Build history of the part. All positions in model axes, mm. A direction names the side the tool comes from. Coordinates: 2 decimals unless noted, no trailing zeros. Write each loop counter-clockwise with the first axis right and the second up, starting at its lowest first coordinate (ties: lowest second). Pieces come first, ordered by that corner, then holes.
Autodesk Fusion 360 part; units mm, degrees
sketch "Sketch1" plane through (0, 0, 0) normal (0, 1, 0) x (1, 0, 0) in component "[a]_belt_clamp_x2"
  line L0 (4.25, 7.875) -> (-4.25, 7.875)
  line L1 (-4.25, 7.875) -> (-4.25, -7.875)
  line L2 (-4.25, -7.875) -> (4.25, -7.875)
  line L3 (4.25, -7.875) -> (4.25, 7.875)
  line L4 (4.25, 7.875) -> (-4.25, -7.875) construction
  line L5 (-4.25, 7.875) -> (4.25, -7.875) construction
  dimension "d1" = 8.5
  dimension "d2" = 15.75
sketch "Sketch2" plane through (0, 0, 0) normal (1, 0, 0) x (0, 1, 0) in component "[a]_belt_clamp_x2"
  line L0 (2.55, 7.875) -> (-3.55, 7.875)
  line L1 (-3.55, 7.875) -> (-3.55, -7.875)
  line L2 (-3.55, -7.875) -> (2.55, -7.875)
  line L3 (2.55, -7.875) -> (2.55, 7.875)
  line L4 (2.55, 7.875) -> (-3.55, -7.875) construction
  line L5 (-3.55, 7.875) -> (2.55, -7.875) construction
  line L6 (-3.55, 4.475) -> (-2.55, 4.475)
  line L7 (0.45, 7.475) -> (0.45, 7.875)
  arc A0 (-2.55, 4.475) -> (0.45, 7.475) centre (-2.55, 7.475) ccw
  line L8 (0, 0) -> (-7.5, 0) construction
  line L9 (-3.55, -4.475) -> (-2.55, -4.475)
  arc A1 (0.45, -7.475) -> (-2.55, -4.475) centre (-2.55, -7.475) ccw
  line L10 (0.45, -7.475) -> (0.45, -7.875)
  point P0 (-0.5, 0)
  dimension "d8" = 6.1
  dimension "d9" = 15.75
  dimension "d10" = 3
  dimension "d11" = 3.4
  dimension "d12" = 3
  dimension "d13" = 1
extrude "Extrude2" add sketch "Sketch2" along normal mid plane 8.6 contours L0 L1 L2 L3 L6 L7 A0 L9 A1 L10 in component "[a]_belt_clamp_x2"
fillet "Fillet1" radius 0.6 2 edges at (0, 0.45, 7.875) (0, 0.45, -7.875) in component "[a]_belt_clamp_x2"
fillet "Fillet2" radius 1 20 edges at (-4.3, -3.05, 4.475) (-4.3, -0.4884, 5.2956) (-4.3, 0.6321, 7.7109) (-4.3, 1.7972, 7.875) (4.3, -3.05, 4.475) (4.3, -0.4884, 5.2956) (4.3, 0.6321, 7.7109) (4.3, 1.7972, 7.875) (-4.3, 1.7972, -7.875) (-4.3, 0.6321, -7.7109) (-4.3, -0.4884, -5.2956) (-4.3, -3.05, -4.475) (4.3, -3.05, -4.475) (4.3, -0.4884, -5.2956) (4.3, 0.6321, -7.7109) (4.3, 1.7972, -7.875) (0, -3.55, 4.475) (-4.3, -3.55, 0) (0, -3.55, -4.475) (4.3, -3.55, 0) in component "[a]_belt_clamp_x2"
hole "Hole1" at (0, -3.55, 0) direction (0, 1, 0) diameter 5 depth 4 tip angle 180 in component "[a]_belt_clamp_x2"
hole "Hole2" at (0, 0.45, 0) direction (0, 1, 0) diameter 3.4 end through all in component "[a]_belt_clamp_x2"
chamfer "Chamfer1" distance 0.4 angle 45 9 edges at (4.0071, 2.55, 7.5821) (0, 2.55, 7.875) (-4.0071, 2.55, 7.5821) (-4.3, 2.55, 0) (-4.0071, 2.55, -7.5821) (0, 2.55, -7.875) (4.0071, 2.55, -7.5821) (4.3, 2.55, 0) (-0.6147, 2.55, 1.585) in component "[a]_belt_clamp_x2"
component "[a]_belt_clamp_x2" placed x (1, 0, 0) y (0, 1, 0) z (0, 0, 1) at (0, 0, 0)
equation "d2 = ab_belt_width * 2 + 3.75 mm"
equation "ab_belt_width = 6 mm"
equation "d9 = ab_belt_width * 2 + 3.75 mm"
equation "d21 = ( 2.5 * 2 ) * 1 mm"
equation "d24 = ( 1.7 * 2 ) * 1 mm"
1. Probe line 1 along X through (y, z) = (0.95, 0); line 2 along X through (y, z) = (-2.2, 0); line 3 along Z through (x, y) = (0, 1.6) (3 decimals). List the from-to ranges inside material, lowest first.
Computed values:
line 1: x = -4.3 to -1.7, 1.7 to 4.3
line 2: x = -4.3 to -2.5, 2.5 to 4.3
line 3: z = -7.875 to -1.7, 1.7 to 7.875
2. 3-axis set-ups, long thin cutter, end or side, ignore diameter. For faces 1 (the face through (-0.05, -3.25, -4.19)), 2 (the face through (2.44, -1.52, 0.54)): which of +Z, -Z, +X, -X, +Y, -Y reach the whole face in a straight line?
Computed values:
face 1: -Z, +X, -X, -Y
face 2: -Y
3. Mould opens along X. For faces 3 (the face through (-0.046, -3.265, 4.174)), 4 (the face through (1, 0.45, -2)), 5 (the face through (-4.3, 0, 0)) say: +X half, -X half, draft (parallel to the pull), parting line (faces both ways), or undercut.
Computed values:
face 3: draft
face 4: undercut
face 5: -X half
4. Saw through at A-A on z = 0. List the corners of the cut face in (x, y).
Computed values:
outline: (-4.3, -2.55) arc R1 ccw to (-3.3, -3.55) - (-2.5, -3.55) - (-2.5, 0.45) - (-1.7, 0.45) - (-1.7, 2.15) - (-2.1, 2.55) - (-3.9, 2.55) - (-4.3, 2.15) - close; (1.7, 0.45) - (2.5, 0.45) - (2.5, -3.55) - (3.3, -3.55) arc R1 ccw to (4.3, -2.55) - (4.3, 2.15) - (3.9, 2.55) - (2.1, 2.55) - (1.7, 2.15) - close
5. Flat gauge pins, fed straight in: pin 1 (1 mm diameter, centred on x = -1, y = -2, fed in from -Z); pin 2 (2.5 mm diameter, centred on x = -1, z = 0, fed in from -Y). Where does each tip first touch, or does it go through?
Computed values:
pin 1: stops at z = -4.66
pin 2: stops at y = 0.45
